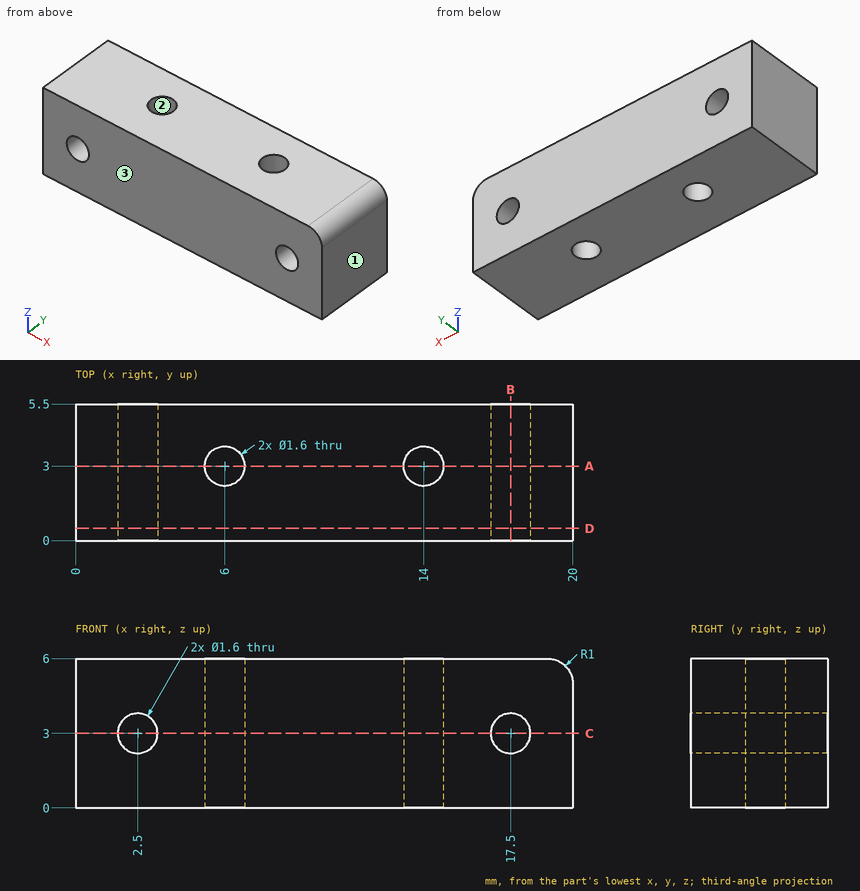
Input: dimensioned drawing with shaded views. Units: mm. Origin: part minimum x, y, z. Round coordinates to 2 decimals unless told otherwise and drop trailing zeros. Order: outer loops, then holes, each group sorted by start corner. A loop starts at its lowest first (then second) coordinate and runs counter-clockwise, first axis right, second up. Notation, with made-up numbers: (77, -27.75) -> (132, -27.75) arc R36 cw to (132, 10.25) -> close; hole circle Ø5 at (10, 62). An arc over 180 degrees is marked (long way). Put each result on its own line as item: value. Start each with the question number.
Q1. Section D-D on y = 0.5. Return the cut outline in (x, z), and give its area (3 significant figures).
Q2. Line query: probe 1 along X at (y, z) = (2.95, 0.7); probe 2 along Z at (x, y) = (2.5, 4); probe 3 along X at (y, z) = (3.6, 0.3). Output: solid intervals per line, ascending.
Q3. Section B-B on x = 17.5. Return the cut outline in (y, z), and give its area (3 significant figures).
Q4. Section A-A on y = 3. Return the cut outline in (x, z), and give its area (3 significant figures).
Q5. Pull-direction query (X, two-part tool) for the marked faces 1, 2 and 3; classes: +X half, -X half, draft (parallel to the pull), parting line (faces both ways), or undercut.
Q6. Section C-C on z = 3. Return the cut outline in (x, y).
Ans:
1. outline: (0, 0) -> (20, 0) -> (20, 5) arc R1 ccw to (19, 6) -> (0, 6) -> close; hole circle Ø1.6 at (2.5, 3); hole circle Ø1.6 at (17.5, 3)
1. area: 116 mm2
2. probe 1: x = 0 to 5.2, 6.8 to 13.2, 14.8 to 20
2. probe 2: z = 0 to 2.2, 3.8 to 6
2. probe 3: x = 0 to 5.47, 6.53 to 13.47, 14.53 to 20
3. outline: (0, 0) -> (5.5, 0) -> (5.5, 2.2) -> (0, 2.2) -> close; (0, 3.8) -> (5.5, 3.8) -> (5.5, 6) -> (0, 6) -> close
3. area: 24.2 mm2
4. outline: (0, 0) -> (5.2, 0) -> (5.2, 6) -> (0, 6) -> close; (6.8, 0) -> (13.2, 0) -> (13.2, 6) -> (6.8, 6) -> close; (14.8, 0) -> (20, 0) -> (20, 5) arc R1 ccw to (19, 6) -> (14.8, 6) -> close; hole circle Ø1.6 at (2.5, 3); hole circle Ø1.6 at (17.5, 3)
4. area: 96.6 mm2
5. face 1: +X half
5. face 2: undercut
5. face 3: draft
6. outline: (0, 0) -> (1.7, 0) -> (1.7, 5.5) -> (0, 5.5) -> close; (3.3, 0) -> (16.7, 0) -> (16.7, 5.5) -> (3.3, 5.5) -> close; (18.3, 0) -> (20, 0) -> (20, 5.5) -> (18.3, 5.5) -> close; hole circle Ø1.6 at (6, 3); hole circle Ø1.6 at (14, 3)
